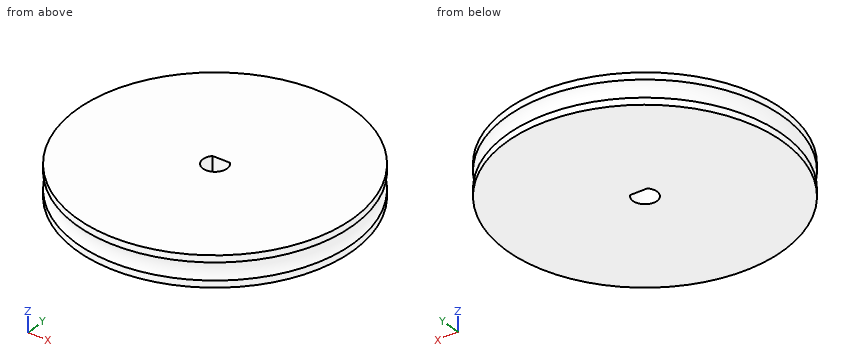
```python
from build123d import *

# Parameters (mm, degrees)
TORUS002_R        = 1.5
BOX084016_W       = 10
BOX084016_H       = 10
BOX084016_DEPTH   = 12
CYLINDER028_R     = 1.57
CYLINDER028_DEPTH = 10
CYLINDER012_R     = 18
CYLINDER012_DEPTH = 4


with BuildPart() as torus002:
    # Torus002 → Torus002 (revolve)
    with BuildSketch(Plane(origin=(0, 0, 2), x_dir=(1, 0, 0), z_dir=(0, -1, 0))):
        with Locations((19, 0)):
            Circle(TORUS002_R)
    revolve(axis=Axis((0, 0, 2), (0, 0, 1)))


with BuildPart() as cube067:
    # Box084016 → Box084016 (new body)
    with BuildSketch(Plane(origin=(-5, 1.1, -1.5), x_dir=(1, 0, 0), z_dir=(0, 0, 1))):
        with Locations((5, 5)):
            Rectangle(BOX084016_W, BOX084016_H)
    extrude(amount=BOX084016_DEPTH)


with BuildPart() as cut057:
    # Cylinder028 → Cylinder028 (new body)
    with BuildSketch(Plane.XY.offset(-1)):
        Circle(CYLINDER028_R)
    extrude(amount=CYLINDER028_DEPTH)

    # Cut057: cut Cube067
    add(cube067.part, mode=Mode.SUBTRACT)


with BuildPart() as cut063:
    # Cylinder012 → Cylinder012 (new body)
    with BuildSketch(Plane.XY):
        Circle(CYLINDER012_R)
    extrude(amount=CYLINDER012_DEPTH)

    # Cut062: cut Cut057
    add(cut057.part, mode=Mode.SUBTRACT)

    # Cut063: cut Torus002
    add(torus002.part, mode=Mode.SUBTRACT)


solid = cut063.part
```
Geometry: final body of the model. Coordinates: model frame, mm. Coordinates: 2 decimals unless noted, no trailing zeros. Order: outer loops, then holes, each group sorted by start corner. A loop starts at its lowest first (then second) coordinate and runs counter-clockwise, first axis right, second up. Notation, with made-up numbers: (13, 7) - (67, 7) arc R11 cw to (67, 14) - close; hole circle Ø1 at (78.5, 30). An arc over 180 degrees is marked (long way). Return JSON: item names as keys, results as strings. Group by question number.
1. Cut plane A-A (y = 0). Output: boundary loops of the cut face in (x, z).
2. Pin query (flat end, axial travel): pin 1 (2 mm diameter, centred on y = 1.5, z = 3, fed in from +X); pin 2 (1 mm diameter, centred on x = -14, z = 1.5, fed in from +Y); pin 3 (0.7 mm diameter, centred on x = -0.5, z = 1.5, fed in from -Y). Return the tip coordinate at first contact, or that it passes through.
3. Cut plane B-B (x = 0). Output: boundary loops of the cut face in (y, z).
4. Cut plane C-C (z = 2.1). Output: boundary loops of the cut face in (x, y), plus the area to 3 significant figures.
5. Material intervals for line 1 along Y through (x, z) = (0, 3.15); line 2 along Y through (x, z) = (0, 1.25); line 3 along X through (y, z) = (0, 1.8), sorted ascending. Write a range as [from, to].
Resolved:
{
 "1": {"outline": "(-18, 0) - (-1.57, 0) - (-1.57, 4) - (-18, 4) - (-18, 3.12) arc R1.5 cw to (-18, 0.88) - close; (1.57, 0) - (18, 0) - (18, 0.88) arc R1.5 cw to (18, 3.12) - (18, 4) - (1.57, 4) - close"},
 "2": {"pin 1": "stops at x = 17.99", "pin 2": "stops at y = 11.38", "pin 3": "stops at y = -17.76"},
 "3": {"outline": "(-18, 0) - (-1.57, 0) - (-1.57, 4) - (-18, 4) - (-18, 3.12) arc R1.5 cw to (-18, 0.88) - close; (1.1, 0) - (18, 0) - (18, 0.88) arc R1.5 cw to (18, 3.12) - (18, 4) - (1.1, 4) - close"},
 "4": {"outline": "circle Ø35.01 at (0, 0); hole (-1.12, 1.1) arc R1.57 ccw (long way) to (1.12, 1.1) - close", "area": "955 mm²"},
 "5": {"line 1": "y = [-18, -1.57], [1.1, 18]", "line 2": "y = [-17.7, -1.57], [1.1, 17.7]", "line 3": "x = [-17.51, -1.57], [1.57, 17.51]"}
}
